For this review, use the dimensioned drawing (mm, ordinates from the lowest corner) and the shaded views. Give positions to 0.01 mm unless a question says otherwise; leave off trailing zeros. Write each loop counter-clockwise with the first axis right and the second up, starting at its lowest first coordinate (ties: lowest second). Pieces come first, ordered by that corner, then holes.
1) For P1, Ø4, axis at x = 3.5, y = 158.5, coming from the +Z side; P2, Ø4, axis at x = 7, z = 53.5, coming from the -Y side; P3, Ø1, axis at x = 6.5, z = 55.5, coming from the -Y side, all flat-tipped, find the tip position at first contact; note any pin that passes through.
2) Wall thickness on line 1 along Y through (x, z) = (3.5, 118) (1 decimal); line 2 along Y through (x, z) = (4.25, 114.5) (1 decimal); line 3 along Z through (x, y) = (5, 110.5) (1 decimal): over which ranges is each line inside the solid? List them lowest first.
3) We need section A-A on z = 46. Give the boundary of the cut face in (x, y).
4) We need section B-B on y = 125. Give the boundary of the cut face in (x, z), and give its area (3 significant figures).
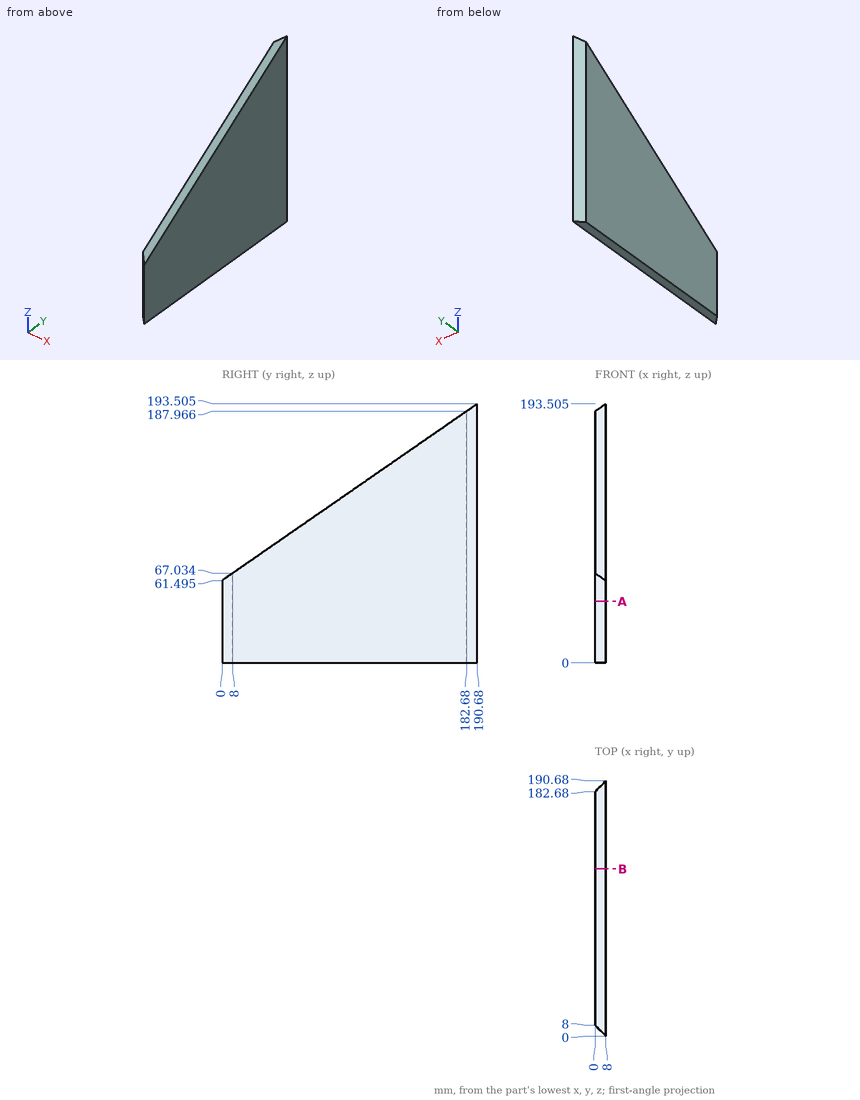
Results list:
1. P1: stops at z = 172.61
1. P2: stops at y = 0
1. P3: stops at y = 1
2. line 1: y = 81.6 to 186.2
2. line 2: y = 76.6 to 186.9
2. line 3: z = 0 to 138
3. outline: (0, 8) - (8, 0) - (8, 190.68) - (0, 182.68) - close
4. outline: (0, 0) - (8, 0) - (8, 148.03) - (0, 148.03) - close
4. area: 1,180 mm2
